Could you check a few things on this model? Use its own coordinates, in mm. A direction names the side the tool comes from. Round coordinates to 2 decimals unless told otherwise and drop trailing zeros. Loops run counter-clockwise (first coordinate to the right, second up) from the corner with the lowest first, then second, coordinate; pieces in that order, holes last. Notation, with made-up numbers: M 60,64 L 101,64 A33 cw 101,99 Z; hole C 86.25,5 d7. An arc over 180 degrees is marked long. One line per item, written item: value. Start each with the question number.
Q1. Imagine slicing it at C-C (x = 0). Please give me the cut outline in (y, z), then the cut area to 3 significant figures.
Q2. Thinking about a two-plate mould opening in X: for faces 1 (the face through (0, 20, 8)), 2 (the face through (0, 25, 5)), 3 (the face through (5, 10, 5)), which applies, released by +X, released by -X, zero draft, split by the parting line, or undercut?
Q3. I'm going to push flat-ended pins straight in: pin 1 Ø2.5 at (x, y) = (-0.5, 0.5) entering from -Z; pin 2 Ø1.5 at (x, y) = (3, 13) entering from -Z. Where does each tip first touch, or does it pass through?
Q4. Imagine slicing it at D-D (y = 10). Please give me the cut outline in (x, z).
Q5. Imagine slicing it at B-B (z = 7.25). Please give me the cut outline in (x, y).
Q6. Please list where these lines run through material, in increasing order: line 1 along Y through (x, z) = (-1, 1); line 2 along Y through (x, z) = (-0.25, 1); line 3 along Z through (x, y) = (-0.75, 17.75).
Q7. Which directions (+Z, -Z, +X, -X, +Y, -Y) give clear straight access to the entire face, cutting with the end or side of a thin tool? Please do faces 4 (the face through (-5, 10, 5)), 5 (the face through (0, 0, 8)).
Q8. Imagine slicing it at A-A (y = 0). Please give me the cut outline in (x, z).
from build123d import *

# Parameters (mm, degrees)
SKETCH_W      = 10
SKETCH_H      = 30
PAD_DEPTH     = 10
SKETCH001_R   = 4
SKETCH001_R_2 = 4.05
SKETCH001_R_3 = 4.1
POCKET_DEPTH  = 8


with BuildPart() as part:
    # Sketch → Pad (new body)
    with BuildSketch(Plane.XY):
        with Locations((0, 10)):
            Rectangle(SKETCH_W, SKETCH_H)
    extrude(amount=PAD_DEPTH)

    # Sketch001 → Pocket (cut)
    with BuildSketch(Plane.XY):
        with Locations((0, 20)):
            Circle(SKETCH001_R)
        with Locations((0, 10)):
            Circle(SKETCH001_R_2)
        Circle(SKETCH001_R_3)
    extrude(amount=POCKET_DEPTH, mode=Mode.SUBTRACT)


solid = part.part
Report:
1. outline: M -5,0 L -4.1,0 L -4.1,8 L 4.1,8 L 4.1,0 L 5.95,0 L 5.95,8 L 14.05,8 L 14.05,0 L 16,0 L 16,8 L 24,8 L 24,0 L 25,0 L 25,10 L -5,10 Z
1. area: 106 mm²
2. face 1: undercut
2. face 2: zero draft
2. face 3: released by +X
3. pin 1: stops at z = 8
3. pin 2: stops at z = 0
4. outline: M -5,0 L -4.05,0 L -4.05,8 L 4.05,8 L 4.05,0 L 5,0 L 5,10 L -5,10 Z
5. outline: M -5,-5 L 5,-5 L 5,25 L -5,25 Z; hole C 0,0 d8.2; hole C 0,10 d8.1; hole C 0,20 d8
6. line 1: y = -5 to -3.98, 3.98 to 6.08, 13.92 to 16.13, 23.87 to 25
6. line 2: y = -5 to -4.09, 4.09 to 5.96, 14.04 to 16.01, 23.99 to 25
6. line 3: z = 8 to 10
7. face 4: +Z, -Z, -X, +Y, -Y
7. face 5: -Z
8. outline: M -5,0 L -4.1,0 L -4.1,8 L 4.1,8 L 4.1,0 L 5,0 L 5,10 L -5,10 Z
